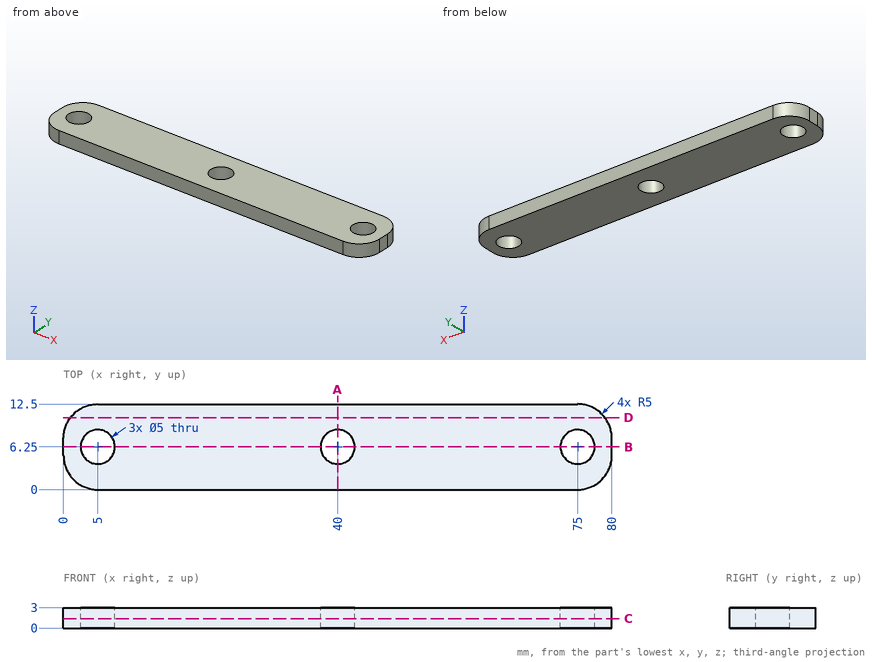
Here's the drawing with two shaded views (mm, measured from the low corner). I have some questions. Round coordinates to 2 decimals unless told otherwise and drop trailing zeros. Write each loop counter-clockwise with the first axis right and the second up, starting at its lowest first coordinate (ties: lowest second). Pieces come first, ordered by that corner, then holes. Notation, with made-up numbers: M 54,4 L 60,4 A18 ccw 60,34 Z; hole C -16,89.5 d3. An arc over 180 degrees is marked long. Use CSV: the item, a comma, the result in double quotes.
(1) Imagine slicing it at A-A (x = 40). Write out the boundary of the cut face in (y, z), plus the area to 3 significant figures.
Check values:
outline,"M 0,0 L 3.75,0 L 3.75,3 L 0,3 Z; M 8.75,0 L 12.5,0 L 12.5,3 L 8.75,3 Z"
area,"22.5 mm^2"
(2) I need wall thicknesses on line 1 along Y through (x, z) = (40, 2.05); line 2 along X through (y, z) = (5.75, 2.3); line 3 along X through (y, z) = (5.25, 2). Which ranges of each line are inside material? Lowest first, please.
Check values:
line 1,"0 to 3.75, 8.75 to 12.5"
line 2,"0 to 2.55, 7.45 to 37.55, 42.45 to 72.55, 77.45 to 80"
line 3,"0 to 2.71, 7.29 to 37.71, 42.29 to 72.71, 77.29 to 80"
(3) Imagine slicing it at C-C (z = 1.4). Write out the boundary of the cut face in (x, y).
Check values:
outline,"M 0,5 A5 ccw 5,0 L 75,0 A5 ccw 80,5 L 80,7.5 A5 ccw 75,12.5 L 5,12.5 A5 ccw 0,7.5 Z; hole C 5,6.25 d5; hole C 40,6.25 d5; hole C 75,6.25 d5"
(4) Imagine slicing it at B-B (y = 6.25). Write out the boundary of the cut face in (x, z).
Check values:
outline,"M 0,0 L 2.5,0 L 2.5,3 L 0,3 Z; M 7.5,0 L 37.5,0 L 37.5,3 L 7.5,3 Z; M 42.5,0 L 72.5,0 L 72.5,3 L 42.5,3 Z; M 77.5,0 L 80,0 L 80,3 L 77.5,3 Z"
(5) Imagine slicing it at D-D (y = 10.5). Write out the boundary of the cut face in (x, z), plus the area to 3 significant figures.
Check values:
outline,"M 1,0 L 79,0 L 79,3 L 1,3 Z"
area,"234 mm^2"
